For this review, take the finished solid that the model builds, in its own axes (mm). Face numbers are marked on the shaded views. A direction names the side the tool comes from. Give positions to 0.01 mm unless a question says otherwise; leave off trailing zeros. Order: outer loops, then holes, each group sorted by start corner. A loop starts at its lowest first (then second) coordinate and runs counter-clockwise, first axis right, second up. Notation, with made-up numbers: M -9.75,-11.5 L -5.75,-11.5 A32 cw -5.75,24.5 Z; hole C 82,-5 d5. An arc over 180 degrees is marked long. Use CSV: the item, a comma, the result in double quotes. Start each with the question number.
(1) Consider section D-D (z = 13). Write out the cut boundary in (x, y).
(2) Tool access review of the marked faces 4, 5 and 6: name each direction out of +Z, -Z, +X, -X, +Y, -Y from which nothing blocks a thin tool from reaching the whole face with its end or side.
(3) Consider section C-C (z = -8.25). Write out the cut boundary in (x, y), and give its area (3 significant figures).
(4) Wall thickness on L1, parallel to Y at x = -9, z = -2.75; L2, parallel to Y at x = -5.25, z = 9; L3, parallel to Z at x = -0.5, y = 2.75: over which ranges is each line inside the solid? List them lowest first. Write a range as from..to.
(5) Consider section B-B (x = -3.5). Write out the cut boundary in (y, z), and give its area (3 significant figures).
(6) Draft analysis for pull direction Z (two halves, no side actions). For the marked faces 1, 2 and 3, state which applies: pulls with the +Z half, pulls with the -Z half, needs draft (parallel to the pull), parting line crosses it, or undercut.
(7) Consider section A-A (y = 0). Write out the cut boundary in (x, z).
(8) Clearance check with flat-ended pins moving along their axes: P1, Ø1.1, axis at y = -3, z = 6.5, coming from the -X side; P2, Ø3, axis at y = 0, z = -6, coming from the -X side; P3, Ø6, axis at x = -8, y = -4, coming from the +Z side; P4, Ø6, axis at y = 2.5, z = -8.5, coming from the -X side. State where each tip first meets the part, or that it passes through.
```python
from build123d import *

# Parameters (mm, degrees)
F1_DEPTH  = 15
F2_R      = 4.25
F2_R_2    = 3.75
F3_DEPTH  = 10
F4_R      = 4.75
F4_R_2    = 4.25
F4_R_3    = 3.75
F5_DEPTH  = 2
F7_DEPTH  = 13
F8_DEPTH  = 2
F7_FACE_W = 10.6
F7_FACE_H = 13
F10_DEPTH = 5
F11_R     = 0.5


with BuildPart() as f1:
    # F0 (on Top) → F1 (new body)
    with BuildSketch(Plane.XY):
        with BuildLine():
            Line((0, 6), (-9, 6))
            ThreePointArc((-9, 6), (-15, 0), (-9, -6))
            Line((-9, -6), (0, -6))
            Line((0, -6), (0, 6))
        make_face()
    extrude(amount=F1_DEPTH)

    # F2 (on Top) → F3 (join)
    with BuildSketch(Plane.XY):
        with Locations((-8.9916, 0)):
            Circle(F2_R)
        with Locations((-8.9916, 0)):
            Circle(F2_R_2, mode=Mode.SUBTRACT)
    extrude(amount=-F3_DEPTH)

    # F4 (on face) → F5 (join)
    with BuildSketch(Plane(origin=(0, 0, -10), x_dir=(1, 0, 0), z_dir=(0, 0, -1))):
        with Locations((-8.9916, 0)):
            Circle(F4_R)
        with Locations((-8.9916, 0)):
            Circle(F4_R_2, mode=Mode.SUBTRACT)
        with Locations((-8.9916, 0)):
            Circle(F4_R_2)
        with Locations((-8.9916, 0)):
            Circle(F4_R_3, mode=Mode.SUBTRACT)
    extrude(amount=F5_DEPTH)

    # F6 (on face) → F7 (cut)
    with BuildSketch(Plane.XY.offset(15)):
        with BuildLine():
            Line((-3, -5.3), (-3, 5.3))
            Line((-3, 5.3), (-9, 5.3))
            ThreePointArc((-9, 5.3), (-14.3, 0), (-9, -5.3))
            Line((-9, -5.3), (-3, -5.3))
        make_face()
    extrude(amount=-F7_DEPTH, mode=Mode.SUBTRACT)

    # F8 (cut, through all): a face of the model
    f8_faces = [f1.faces().sort_by_distance(p)[0] for p in [
        (-8.9916, 0, 0),
    ]]
    extrude(f8_faces, amount=-F8_DEPTH, mode=Mode.SUBTRACT)

    # F9 (on face) + F7_face (on face) → F10 (cut)
    with BuildSketch(Plane.YZ):
        with BuildLine():
            Line((-3.5, 4.6132088465), (-3.5, 2.6055402327))
            ThreePointArc((-3.5, 2.6055402327), (-3.3226413721, 2.1773586279), (-2.8944597673, 2))
            Line((-2.8944597673, 2), (0, 2))
            Line((0, 2), (2.8944597673, 2))
            ThreePointArc((2.8944597673, 2), (3.3226413721, 2.1773586279), (3.5, 2.6055402327))
            Line((3.5, 2.6055402327), (3.5, 4.6132088465))
            ThreePointArc((3.5, 4.6132088465), (3.5269042645, 4.7917008345), (3.6052263353, 4.9543319584))
            Line((3.6052263353, 4.9543319584), (4.8947736647, 6.8456680416))
            ThreePointArc((4.8947736647, 6.8456680416), (4.9730957355, 7.0082991655), (5, 7.1867911535))
            Line((5, 7.1867911535), (5, 11.5944597673))
            ThreePointArc((5, 11.5944597673), (4.8226413721, 12.0226413721), (4.3944597673, 12.2))
            Line((4.3944597673, 12.2), (4.0912942222, 12.2))
            ThreePointArc((4.0912942222, 12.2), (3.668239264, 12.0277073591), (3.4859255549, 11.608873307))
            Line((3.4859255549, 11.608873307), (3.4140744451, 8.591126693))
            ThreePointArc((3.4140744451, 8.591126693), (3.231760736, 8.1722926409), (2.8087057778, 8))
            Line((2.8087057778, 8), (2.3789951326, 8))
            ThreePointArc((2.3789951326, 8), (1.9270666838, 8.2025022065), (1.7774022402, 8.6745689611))
            Line((1.7774022402, 8.6745689611), (2.5, 14.9720872054))
            Line((2.5, 14.9720872054), (2.503202805, 15))
            Line((2.503202805, 15), (-2.5090757857, 15))
            Line((-2.5090757857, 15), (-2.5, 14.9720872054))
            Line((-2.5, 14.9720872054), (-1.7774022402, 8.6745689611))
            ThreePointArc((-1.7774022402, 8.6745689611), (-1.9270666838, 8.2025022065), (-2.3789951326, 8))
            Line((-2.3789951326, 8), (-2.8087057778, 8))
            ThreePointArc((-2.8087057778, 8), (-3.231760736, 8.1722926409), (-3.4140744451, 8.591126693))
            Line((-3.4140744451, 8.591126693), (-3.4859255549, 11.608873307))
            ThreePointArc((-3.4859255549, 11.608873307), (-3.668239264, 12.0277073591), (-4.0912942222, 12.2))
            Line((-4.0912942222, 12.2), (-4.3944597673, 12.2))
            ThreePointArc((-4.3944597673, 12.2), (-4.8226413721, 12.0226413721), (-5, 11.5944597673))
            Line((-5, 11.5944597673), (-5, 7.1867911535))
            ThreePointArc((-5, 7.1867911535), (-4.9730957355, 7.0082991655), (-4.8947736647, 6.8456680416))
            Line((-4.8947736647, 6.8456680416), (-3.6052263353, 4.9543319584))
            ThreePointArc((-3.6052263353, 4.9543319584), (-3.5269042645, 4.7917008345), (-3.5, 4.6132088465))
        make_face()
    with BuildSketch(Plane(origin=(-3, 0, 8.5), x_dir=(0, -1, 0), z_dir=(-1, 0, 0))):
        Rectangle(F7_FACE_W, F7_FACE_H)
    extrude(amount=-F10_DEPTH, dir=(1, 0, 0), mode=Mode.SUBTRACT)

    # F11
    f11_edges = [f1.edges().sort_by_distance(p)[0] for p in [
        (-13.7416, 0, -12),
    ]]
    fillet(f11_edges, radius=F11_R)


solid = f1.part
```
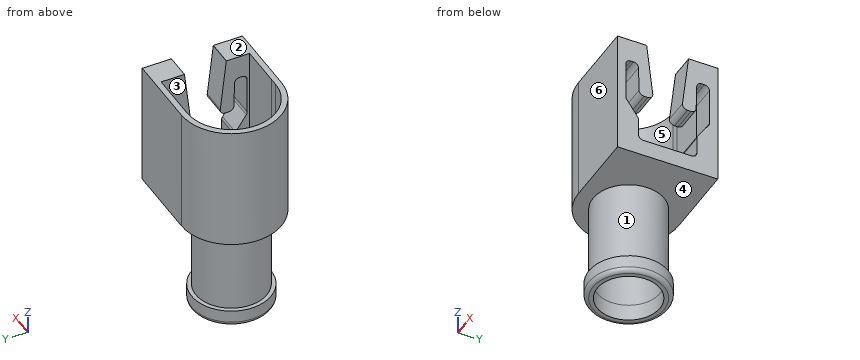
Check result:
1,outline,"M -9,-6 L 0,-6 L 0,-2.27 L -3,-2.27 L -3,-5.3 L -9,-5.3 A5.3 cw -9,5.3 L -3,5.3 L -3,2.27 L 0,2.27 L 0,6 L -9,6 A6 ccw Z"
2,face 4,"none"
2,face 5,"+Z"
2,face 6,"+Z, -Z, +X, -X, -Y"
3,outline,"C -8.99,0 d8.5; hole C -8.99,0 d7.5"
3,area,"12.6 mm^2"
4,L1,"y = -4.25..-3.75, 3.75..4.25"
4,L2,"y = -6..-5.3, 5.3..6"
4,L3,"z = 0..2, 8..15"
5,outline,"M -6,0 L 6,0 L 6,15 L 5.3,15 L 5.3,2 L -5.3,2 L -5.3,15 L -6,15 Z"
5,area,"42.2 mm^2"
6,face 1,"undercut"
6,face 2,"pulls with the +Z half"
6,face 3,"needs draft"
7,outline,"M -15,0 L -13.24,0 L -13.24,-10 L -13.74,-10 L -13.74,-11.5 A0.5 ccw -13.24,-12 L -12.74,-12 L -12.74,2 L -14.3,2 L -14.3,15 L -15,15 Z; M -5.24,-12 L -4.74,-12 A0.5 ccw -4.24,-11.5 L -4.24,-10 L -4.74,-10 L -4.74,0 L 0,0 L 0,2 L -5.24,2 Z"
8,P1,"stops at x = -14.48"
8,P2,"stops at x = -13.24"
8,P3,"stops at z = 15"
8,P4,"stops at x = -13.74"
